Source: CAD feature listing. Evaluate the final solid. Frame: model axes, mm. A direction names the side the tool comes from. Coordinates: 2 decimals unless noted, no trailing zeros. Write each loop counter-clockwise with the first axis right and the second up, starting at its lowest first coordinate (ties: lowest second). Pieces come first, ordered by that corner, then holes. Notation, with made-up numbers: M 5.5,38.5 L 44.5,38.5 A25 cw 44.5,64.5 Z; hole C -6,89 d5. An arc over 180 degrees is marked long. Answer as CSV lines item,"result". Start each with the question number.
1. Contact query for flat-ended pins moving along their axis: pin 1 Ø24 at (x, y) = (551.5, 124.5) entering from +Z; pin 2 Ø9 at (x, y) = (-555, -530) entering from +Z. Output: stop coordinate, or through.
2. Mould query, pull axis Y, two halves, no side actions, for faces 4 (the face through (-9, 276.135, 10)), 5 (the face through (-285, -75, 108)). Classes: pulls with the +Y half, pulls with the -Y half, needs draft (parallel to the pull), parting line crosses it, or undercut.
3. Section A-A on y = -268. Return the cut outline in (x, z), plus the area to 3 significant figures.
4. Section B-B on z = 42.5. Return the cut outline in (x, y).
5. Reachability of faces 1 (the face through (-41.376, -161, 63)), 2 (the face through (-9, 187, 127)), 3 (the face through (-546, -399, 97)) from +Z, -Z, +X, -X, +Y, -Y: full face, straight path, thin tool, end or side. Return the list, or none.
6. Line query: probe 1 along X at (y, z) = (-127.5, 88); probe 2 along X at (y, z) = (-424, 22); probe 3 along X at (y, z) = (-158, 17.5). Output: solid intervals per line, ascending. Write a range as [from, to].
7. Section D-D on x = 342. Count the separate pieces of the cut face and the enclosed holes in it, plus the area to 3 significant figures.
8. Section C-C on y = 50.5. Return the cut outline in (x, z).
```python
from build123d import *

# Parameters (mm, degrees)
F0_W     = 1140
F0_H     = 980
F1_DEPTH = 127
F2_W     = 480
F2_H     = 89
F2_W_2   = 520
F3_DEPTH = 980.001
F4_W     = 30
F4_H     = 30
F5_DEPTH = 1140.001
F6_W     = 1020
F6_H     = 860
F7_DEPTH = 25


with BuildPart() as f1:
    # F0 (on Top) → F1 (new body)
    with BuildSketch(Plane.XY):
        with Locations((-1.375834, -153.865348)):
            Rectangle(F0_W, F0_H)
    extrude(amount=F1_DEPTH)

    # F2 (on face) → F3 (cut, through all)
    with BuildSketch(Plane.XZ.offset(643.865348)):
        with Locations((-281.375834, 63.5)):
            Rectangle(F2_W, F2_H)
        with Locations((258.624166, 63.5)):
            Rectangle(F2_W_2, F2_H)
    extrude(amount=-F3_DEPTH, mode=Mode.SUBTRACT)

    # F4 (on face) → F5 (cut, through all)
    with BuildSketch(Plane.YZ.offset(568.624166)):
        with Locations((-528.865348, 112)):
            Rectangle(F4_W, F4_H)
        Polygon((266.134652, 127), (236.134652, 127), (236.134652, 97), (236.134652, 95.564112), (266.134652, 95.564112), align=None)
        with Locations((-398.865348, 112)):
            Rectangle(F4_W, F4_H)
        with Locations((-268.865348, 112)):
            Rectangle(F4_W, F4_H)
        with Locations((-138.865348, 112)):
            Rectangle(F4_W, F4_H)
        with Locations((-8.865348, 112)):
            Rectangle(F4_W, F4_H)
        with Locations((121.134652, 112)):
            Rectangle(F4_W, F4_H)
    extrude(amount=-F5_DEPTH, mode=Mode.SUBTRACT)

    # F6 (on face) → F7 (cut)
    with BuildSketch(Plane(origin=(0, 0, 0), x_dir=(1, 0, 0), z_dir=(0, 0, -1))):
        with Locations((-1.375834, 153.865348)):
            Rectangle(F6_W, F6_H)
    extrude(amount=-F7_DEPTH, mode=Mode.SUBTRACT)


solid = f1.part
```
Values:
1,pin 1,"z = 127"
1,pin 2,"z = 97"
2,face 4,"undercut"
2,face 5,"needs draft"
3,outline,"M -571.38,0 L -511.38,0 L -511.38,19 L -521.38,19 L -521.38,97 L -571.38,97 Z; M -41.38,25 L -1.38,25 L -1.38,97 L -41.38,97 Z; M 508.62,0 L 568.62,0 L 568.62,97 L 518.62,97 L 518.62,19 L 508.62,19 Z"
3,area,"13,000 mm²"
4,outline,"M -571.38,-643.87 L -521.38,-643.87 L -521.38,336.13 L -571.38,336.13 Z; M -41.38,-643.87 L -1.38,-643.87 L -1.38,336.13 L -41.38,336.13 Z; M 518.62,-643.87 L 568.62,-643.87 L 568.62,336.13 L 518.62,336.13 Z"
5,face 1,"+Y, -Y"
5,face 2,"+Z, +X, -X, +Y, -Y"
5,face 3,"+Z, +X, -X"
6,probe 1,"[-571.38, -521.38], [-41.38, -1.38], [518.62, 568.62]"
6,probe 2,"[-571.38, -521.38], [518.62, 568.62]"
6,probe 3,"[-571.38, -511.38], [508.62, 568.62]"
7,separate pieces,"10"
7,enclosed holes,"0"
7,area,"16,900 mm²"
8,outline,"M -571.38,0 L -511.38,0 L -511.38,19 L -521.38,19 L -521.38,108 L -41.38,108 L -41.38,25 L -1.38,25 L -1.38,108 L 518.62,108 L 518.62,19 L 508.62,19 L 508.62,0 L 568.62,0 L 568.62,127 L -571.38,127 Z"
